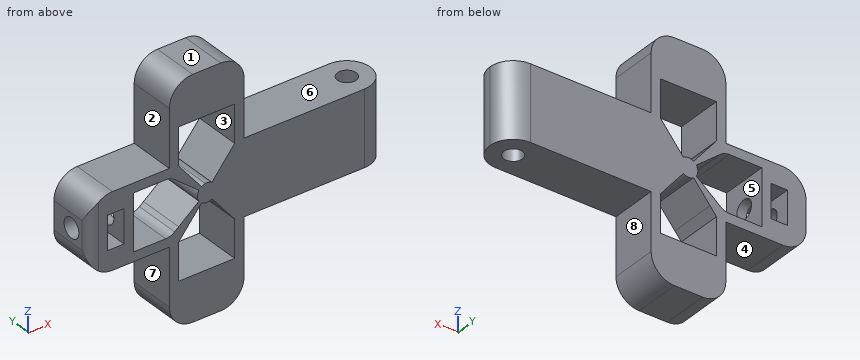
from build123d import *

# Parameters (mm, degrees)
F0_R      = 2
F1_DEPTH  = 16
F2_W      = 3.5
F2_H      = 7.2
F3_DEPTH  = 5
F4_DEPTH  = 5
F6_R      = 2.1
F7_DEPTH  = 10
F8_R      = 3
F9_DEPTH  = 5
F10_DEPTH = 5
F11_DEPTH = 5
F12_DEPTH = 5
F13_R     = 5


with BuildPart() as f1:
    # F0 (on Top) → F1 (new body)
    with BuildSketch(Plane.XY):
        with BuildLine():
            ThreePointArc((32, 0), (30.5355339059, 3.5355339059), (27, 5))
            Line((27, 5), (18, 5))
            Line((18, 5), (8, 5))
            Line((8, 5), (-32, 5))
            Line((-32, 5), (-32, -3))
            Line((-32, -3), (-30, -3))
            Line((-30, -3), (-30, -5))
            Line((-30, -5), (27, -5))
            ThreePointArc((27, -5), (30.5355339059, -3.5355339059), (32, 0))
        make_face()
        with Locations((27, 0)):
            Circle(F0_R, mode=Mode.SUBTRACT)
        with BuildLine():
            ThreePointArc((-32, -3), (-31.4142135624, -4.4142135624), (-30, -5))
            Line((-30, -5), (-30, -3))
            Line((-30, -3), (-32, -3))
        make_face()
    extrude(amount=F1_DEPTH)

    # F2 (on Front) → F3 (cut)
    with BuildSketch(Plane.XZ):
        with BuildLine():
            Line((-32, 16), (-32, 11))
            ThreePointArc((-32, 11), (-30.5355339059, 14.5355339059), (-27, 16))
            Line((-27, 16), (-32, 16))
        make_face()
        with BuildLine():
            Line((-32, 0), (-27, 0))
            ThreePointArc((-27, 0), (-30.5355339059, 1.4644660941), (-32, 5))
            Line((-32, 5), (-32, 0))
        make_face()
        with Locations((-26.25, 8)):
            Rectangle(F2_W, F2_H)
        with BuildLine():
            Line((-22.5, 2), (-14.5, 2))
            Line((-14.5, 2), (-12.8, 3.3783783784))
            Line((-12.8, 3.3783783784), (-8.4655588505, 6.8927901212))
            ThreePointArc((-8.4655588505, 6.8927901212), (-8.8, 8), (-8.4655588505, 9.1072098788))
            Line((-8.4655588505, 9.1072098788), (-12.8, 12.6216216216))
            Line((-12.8, 12.6216216216), (-14.5, 14))
            Line((-14.5, 14), (-22.5, 14))
            Line((-22.5, 14), (-22.5, 2))
        make_face()
    extrude(amount=-F3_DEPTH, mode=Mode.SUBTRACT)

    # F2 (on Front) → F4 (cut)
    with BuildSketch(Plane.XZ):
        with Locations((-26.25, 8)):
            Rectangle(F2_W, F2_H)
        with BuildLine():
            Line((-22.5, 2), (-14.5, 2))
            Line((-14.5, 2), (-12.8, 3.3783783784))
            Line((-12.8, 3.3783783784), (-8.4655588505, 6.8927901212))
            ThreePointArc((-8.4655588505, 6.8927901212), (-8.8, 8), (-8.4655588505, 9.1072098788))
            Line((-8.4655588505, 9.1072098788), (-12.8, 12.6216216216))
            Line((-12.8, 12.6216216216), (-14.5, 14))
            Line((-14.5, 14), (-22.5, 14))
            Line((-22.5, 14), (-22.5, 2))
        make_face()
        with BuildLine():
            Line((-32, 16), (-32, 11))
            ThreePointArc((-32, 11), (-30.5355339059, 14.5355339059), (-27, 16))
            Line((-27, 16), (-32, 16))
        make_face()
        with BuildLine():
            Line((-32, 0), (-27, 0))
            ThreePointArc((-27, 0), (-30.5355339059, 1.4644660941), (-32, 5))
            Line((-32, 5), (-32, 0))
        make_face()
    extrude(amount=F4_DEPTH, mode=Mode.SUBTRACT)

    # F6 (on offset) → F7 (cut)
    with BuildSketch(Plane.YZ.offset(-32)):
        with Locations((0, 8)):
            Circle(F6_R)
    extrude(amount=F7_DEPTH, mode=Mode.SUBTRACT)

    # F8
    f8_edges = [f1.edges().sort_by_distance(p)[0] for p in [
        (-14.5, 0, 2),
        (-14.5, 0, 14),
    ]]
    fillet(f8_edges, radius=F8_R)

    # F2 (on Front) → F9 (join)
    with BuildSketch(Plane.XZ):
        Polygon((-14.8, 33.2), (-14.8, 16), (-12.8, 16), (-12.8, 23.7), (-0.8, 23.7), (-0.8, 16), (1.2, 16), (1.2, 33.2), align=None)
        Polygon((-12.8, 0), (-14.8, 0), (-14.8, -17.2), (1.2, -17.2), (1.2, 0), (-0.8, 0), (-0.8, -7.7), (-12.8, -7.7), align=None)
    extrude(amount=F9_DEPTH)

    # F2 (on Front) → F10 (join)
    with BuildSketch(Plane.XZ):
        Polygon((-14.8, 33.2), (-14.8, 16), (-12.8, 16), (-12.8, 23.7), (-0.8, 23.7), (-0.8, 16), (1.2, 16), (1.2, 33.2), align=None)
        Polygon((-12.8, 0), (-14.8, 0), (-14.8, -17.2), (1.2, -17.2), (1.2, 0), (-0.8, 0), (-0.8, -7.7), (-12.8, -7.7), align=None)
    extrude(amount=-F10_DEPTH)

    # F2 (on Front) → F11 (cut)
    with BuildSketch(Plane.XZ):
        with BuildLine():
            Line((-12.8, 0.3), (-12.8, 0))
            Line((-12.8, 0), (-0.8, 0))
            Line((-0.8, 0), (-0.8, 0.3))
            Line((-0.8, 0.3), (-5.6927901212, 6.3344411495))
            ThreePointArc((-5.6927901212, 6.3344411495), (-6.3673294485, 6.047361735), (-7.1, 6.0226280067))
            Line((-7.1, 6.0226280067), (-7.1, 2))
            Line((-7.1, 2), (-11.4216216216, 2))
            Line((-11.4216216216, 2), (-12.8, 0.3))
        make_face()
        with BuildLine():
            Line((-7.9072098788, 6.3344411495), (-11.4216216216, 2))
            Line((-11.4216216216, 2), (-7.1, 2))
            Line((-7.1, 2), (-7.1, 6.0226280067))
            ThreePointArc((-7.1, 6.0226280067), (-7.5206710552, 6.1343544736), (-7.9072098788, 6.3344411495))
        make_face()
        with BuildLine():
            Line((-0.8, 16), (-12.8, 16))
            Line((-12.8, 16), (-12.8, 15.7))
            Line((-12.8, 15.7), (-11.4216216216, 14))
            Line((-11.4216216216, 14), (-7.1, 14))
            Line((-7.1, 14), (-7.1, 9.9773719933))
            ThreePointArc((-7.1, 9.9773719933), (-6.3673294485, 9.952638265), (-5.6927901212, 9.6655588505))
            Line((-5.6927901212, 9.6655588505), (-0.8, 15.7))
            Line((-0.8, 15.7), (-0.8, 16))
        make_face()
        with BuildLine():
            Line((-7.1, 14), (-11.4216216216, 14))
            Line((-11.4216216216, 14), (-7.9072098788, 9.6655588505))
            ThreePointArc((-7.9072098788, 9.6655588505), (-7.5206710552, 9.8656455264), (-7.1, 9.9773719933))
            Line((-7.1, 9.9773719933), (-7.1, 14))
        make_face()
    extrude(amount=-F11_DEPTH, mode=Mode.SUBTRACT)

    # F2 (on Front) → F12 (cut)
    with BuildSketch(Plane.XZ):
        with BuildLine():
            Line((-12.8, 0.3), (-12.8, 0))
            Line((-12.8, 0), (-0.8, 0))
            Line((-0.8, 0), (-0.8, 0.3))
            Line((-0.8, 0.3), (-5.6927901212, 6.3344411495))
            ThreePointArc((-5.6927901212, 6.3344411495), (-6.3673294485, 6.047361735), (-7.1, 6.0226280067))
            Line((-7.1, 6.0226280067), (-7.1, 2))
            Line((-7.1, 2), (-11.4216216216, 2))
            Line((-11.4216216216, 2), (-12.8, 0.3))
        make_face()
        with BuildLine():
            Line((-7.9072098788, 6.3344411495), (-11.4216216216, 2))
            Line((-11.4216216216, 2), (-7.1, 2))
            Line((-7.1, 2), (-7.1, 6.0226280067))
            ThreePointArc((-7.1, 6.0226280067), (-7.5206710552, 6.1343544736), (-7.9072098788, 6.3344411495))
        make_face()
        with BuildLine():
            Line((-0.8, 16), (-12.8, 16))
            Line((-12.8, 16), (-12.8, 15.7))
            Line((-12.8, 15.7), (-11.4216216216, 14))
            Line((-11.4216216216, 14), (-7.1, 14))
            Line((-7.1, 14), (-7.1, 9.9773719933))
            ThreePointArc((-7.1, 9.9773719933), (-6.3673294485, 9.952638265), (-5.6927901212, 9.6655588505))
            Line((-5.6927901212, 9.6655588505), (-0.8, 15.7))
            Line((-0.8, 15.7), (-0.8, 16))
        make_face()
        with BuildLine():
            Line((-7.1, 14), (-11.4216216216, 14))
            Line((-11.4216216216, 14), (-7.9072098788, 9.6655588505))
            ThreePointArc((-7.9072098788, 9.6655588505), (-7.5206710552, 9.8656455264), (-7.1, 9.9773719933))
            Line((-7.1, 9.9773719933), (-7.1, 14))
        make_face()
    extrude(amount=F12_DEPTH, mode=Mode.SUBTRACT)

    # F13
    f13_edges = [f1.edges().sort_by_distance(p)[0] for p in [
        (-14.8, 0, 33.2),
        (1.2, 0, 33.2),
        (-14.8, 0, -17.2),
        (1.2, 0, -17.2),
    ]]
    fillet(f13_edges, radius=F13_R)


solid = f1.part
Work out the finished part from the listing and answer in its coordinate system (mm). Face numbers are marked on the shaded views. A direction names the side the tool comes from. Round coordinates to 2 decimals unless told otherwise and drop trailing zeros. Order: outer loops, then holes, each group sorted by start corner. A loop starts at its lowest first (then second) coordinate and runs counter-clockwise, first axis right, second up. Notation, with made-up numbers: M 12.25,42.25 L 21.25,42.25 A28 ccw 21.25,62.25 Z; hole C 48,33.5 d3. An arc over 180 degrees is marked long. Put each result on its own line as item: value. Start each with the question number.
Q1. A tool of negligible diameter and unlimited length cuts with its end or side. For the marked faces 5, 6, 7 and 8, from which of +Z, -Z, +X, -X, +Y, -Y can it reach the whole face along a straight path? Write none if from no direction.
Q2. For a pull along Z with two mould halves and no side action, classify the marked faces 1, 2, 3 and 4 as pulls with the +Z half, pulls with the -Z half, needs draft (parallel to the pull), parting line crosses it, or undercut.
Q3. Section A-A, the plane z = 8 is taken. Write down the section's boundary in (x, y).
Q4. Section D-D, the plane y = -0.75 is taken. Give the number of separate pieces and of enclosed holes in the cut face, and give its area (3 significant figures).
Q5. Section C-C, the plane z = -7 is taken. Write down the section's boundary in (x, y), and give its area (3 significant figures).
Q6. Section B-B, the plane x = -2 is taken. Write down the section's boundary in (y, z).
Q7. Flat-ended cylindrical pins translate along their axes: pin 1 (3 mm diameter, centred on y = 0.5, z = 21.5, fed in from +X); pin 2 (3.5 mm diameter, centred on x = -18.5, y = -1, fed in from -Z); pin 3 (4 mm diameter, centred on x = -25.5, y = -1, fed in from +Z). Find the tip coordinate at first contact, or state that the pin passes through.
Q8. Straight lines are drawn through the part: L1, parallel to Z at x = -23.4, y = 0; L2, parallel to Z at x = -27, y = -3.25; L3, parallel to Y at x = -24, z = 8. For each, find the intervals that lie inside material, in ascending order. Write a range as [from, to].
Findings below:
1. face 5: +Y, -Y
1. face 6: +Z, +X, +Y, -Y
1. face 7: -Z, -X, +Y, -Y
1. face 8: -Z, +X, +Y, -Y
2. face 1: pulls with the +Z half
2. face 2: needs draft
2. face 3: undercut
2. face 4: pulls with the -Z half
3. outline: M -32,-3 A2 ccw -30,-5 L -28,-5 L -28,-2.1 L -32,-2.1 Z; M -32,2.1 L -28,2.1 L -28,5 L -32,5 Z; M -24.5,-5 L -22.5,-5 L -22.5,-2.1 L -24.5,-2.1 Z; M -24.5,2.1 L -22.5,2.1 L -22.5,5 L -24.5,5 Z; M -8.8,-5 L 27,-5 A5 ccw 27,5 L -8.8,5 Z; hole C 27,0 d4
4. separate pieces: 2
4. enclosed holes: 2
4. area: 1,020 mm^2
5. outline: M -14.8,-5 L -12.8,-5 L -12.8,5 L -14.8,5 Z; M -0.8,-5 L 1.2,-5 L 1.2,5 L -0.8,5 Z
5. area: 40.0 mm^2
6. outline: M -5,-16.86 L 5,-16.86 L 5,-7.7 L -5,-7.7 Z; M -5,1.78 L 5,1.78 L 5,14.22 L -5,14.22 Z; M -5,23.7 L 5,23.7 L 5,32.86 L -5,32.86 Z
7. pin 1: stops at x = 1.2
7. pin 2: stops at z = 0
7. pin 3: stops at z = 16
8. L1: z = [0, 5.9], [10.1, 16]
8. L2: z = [0, 4.4], [11.6, 16]
8. L3: y = [-5, -2.1], [2.1, 5]
